Build history of the part. All positions in model axes, mm. Round coordinates to 2 decimals unless told otherwise and drop trailing zeros. Loops run counter-clockwise (first coordinate to the right, second up) from the corner with the lowest first, then second, coordinate; pieces in that order, holes last. Notation, with made-up numbers: M 13,-37 L 51,-37 A33 cw 51,-6 Z; hole C 49.25,44.5 d6. An arc over 180 degrees is marked long. Write each question's results on one line, items separated by ' | '. Start each with the question number.
```python
from build123d import *

# Parameters (mm, degrees)
SKETCH_R        = 20
PAD_DEPTH       = 1.6
SKETCH001_W     = 16
SKETCH001_H     = 27
PAD001_DEPTH    = 1.6
FILLET_R        = 0.4
SKETCH002_R     = 11.629701
POCKET_DEPTH    = 0.001
POCKET001_DEPTH = 1.601


with BuildPart() as part:
    # Sketch → Pad (new body)
    with BuildSketch(Plane.XY):
        Circle(SKETCH_R)
    extrude(amount=PAD_DEPTH)

    # Sketch001 → Pad001 (join)
    with BuildSketch(Plane.XY):
        with Locations((0, -13.5)):
            Rectangle(SKETCH001_W, SKETCH001_H)
    extrude(amount=PAD001_DEPTH)

    # Fillet
    fillet_edges = [part.edges().sort_by_distance(p)[0] for p in [
        (0, -27, 1.6),
        (0, -27, 0),
    ]]
    fillet(fillet_edges, radius=FILLET_R)

    # Sketch002 → Pocket (cut, through all)
    with BuildSketch(Plane.XY):
        Circle(SKETCH002_R)
    extrude(amount=-POCKET_DEPTH, mode=Mode.SUBTRACT)

    # Sketch002 → Pocket001 (cut, through all)
    with BuildSketch(Plane.XY):
        Circle(SKETCH002_R)
    extrude(amount=POCKET001_DEPTH, mode=Mode.SUBTRACT)


solid = part.part
```
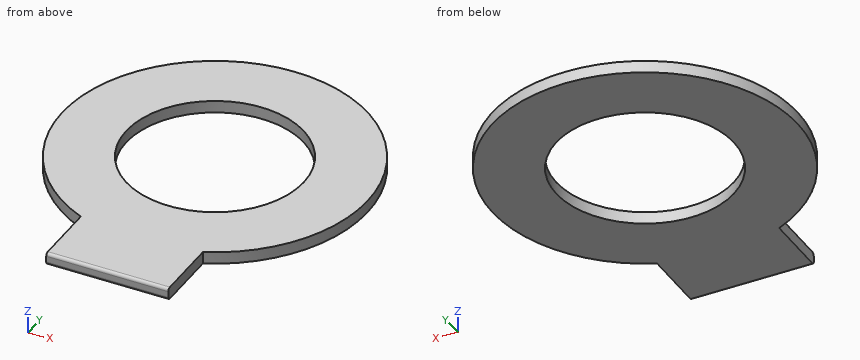
Item 1: Drill centre lines: line 1 along X through (y, z) = (0, 1.1); line 2 along Y through (x, z) = (0, 1.05); line 3 along Y through (x, z) = (10.5, 0.9). Where is each one in solid material? Low to high. Write a range as [from, to].
Item 2: Saw through at D-D, the plane y = -22. Give the cut face in (x, z).
Item 3: Saw through at C-C, the plane y = -9. Give the cut face in (x, z), then the cut area to 3 significant figures.
Item 4: Saw through at A-A, the plane x = 0. Give the cut face in (y, z).
Item 5: Saw through at B-B, the plane y = 0. Give the cut face in (x, z), then the cut area to 3 significant figures.
Item 6: Drop a flat-ended pin along its axis: pin 1 (0.8 mm diameter, centred on y = -22.5, z = 1, fed in from +X). Give the stop position or say it passes through.
Working result:
1) line 1: x = [-20, -11.63], [11.63, 20] | line 2: y = [-27, -11.63], [11.63, 20] | line 3: y = [-17.02, -5], [5, 17.02]
2) outline: M -8,0 L 8,0 L 8,1.6 L -8,1.6 Z
3) outline: M -17.86,0 L -7.37,0 L -7.37,1.6 L -17.86,1.6 Z; M 7.37,0 L 17.86,0 L 17.86,1.6 L 7.37,1.6 Z | area: 33.6 mm²
4) outline: M -27,0.4 A0.4 ccw -26.6,0 L -11.63,0 L -11.63,1.6 L -26.6,1.6 A0.4 ccw -27,1.2 Z; M 11.63,0 L 20,0 L 20,1.6 L 11.63,1.6 Z
5) outline: M -20,0 L -11.63,0 L -11.63,1.6 L -20,1.6 Z; M 11.63,0 L 20,0 L 20,1.6 L 11.63,1.6 Z | area: 26.8 mm²
6) pin 1: stops at x = 8
